Could you check a few things on this drawing? It's one solid part, dimensions in mm from its lowest x, y, z. A direction names the side the tool comes from. Round coordinates to 2 decimals unless told otherwise and drop trailing zeros. Loops run counter-clockwise (first coordinate to the right, second up) from the corner with the lowest first, then second, coordinate; pieces in that order, holes last. Notation, with made-up numbers: M 85.5,-24.5 L 132.5,-24.5 A10 cw 132.5,-10.5 Z; hole C 23,51 d1. An arc over 180 degrees is marked long. Write item = value, one per line. Start each with the question number.
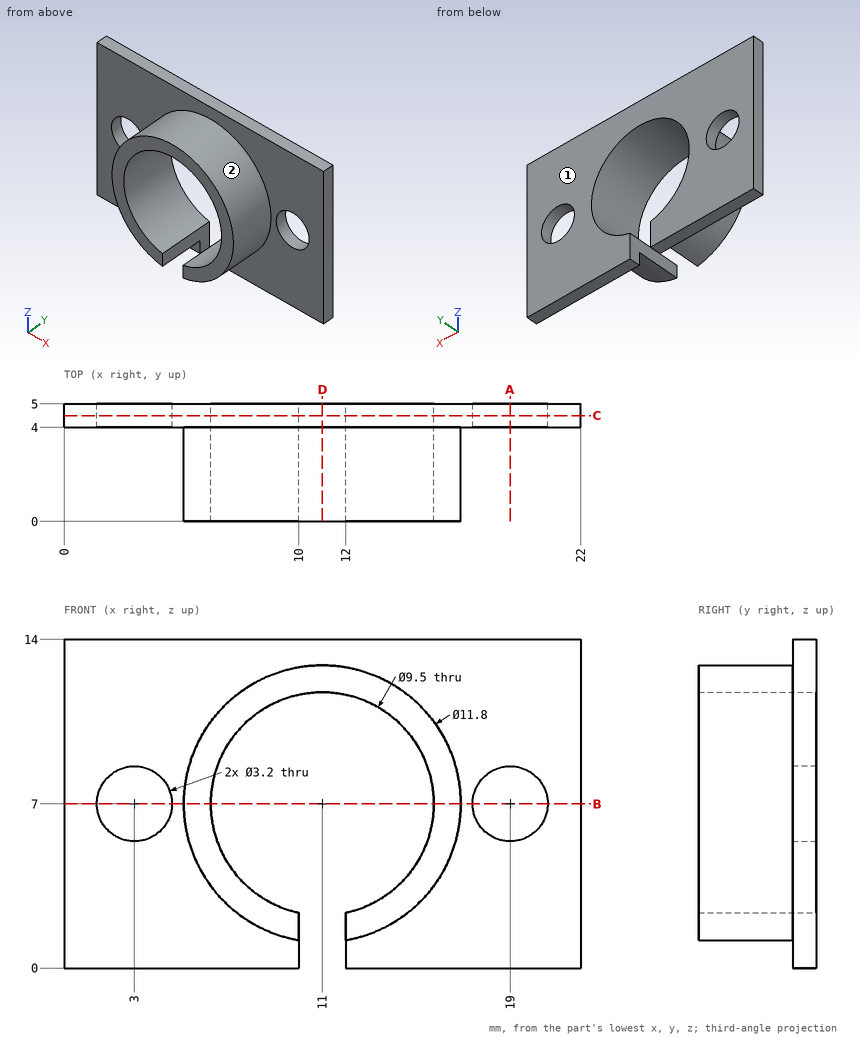
Item 1: For the marked faces 1 and 2, which set-ups out of +Z, -Z, +X, -X, +Y, -Y let a thin tool reach every point of the face, with its end or its side?
Item 2: I want a section at B-B, the plane z = 7. List the corners of the cut face in (x, y) for me.
Item 3: Please list where these lines run through material, in increasing order: line 1 (X direction, y = 4.85, z = 7); line 2 (X direction, y = 4.2, z = 5.75); line 3 (Y direction, x = 11, z = 13.5). Write a range as [from, to].
Item 4: I want a section at C-C, the plane y = 4.5. List the corners of the cut face in (x, z) for me, then the cut area to 3 significant figures.
Item 5: I want a section at D-D, the plane x = 11. List the corners of the cut face in (y, z) for me, then the cut area to 3 significant figures.
Item 6: Will these pins go through, and if not, where does the flat tip stop? pin 1 Ø1 at (x, z) = (18, 6) entering from +Y; pin 2 Ø1 at (x, z) = (4.5, 2) entering from -Y; pin 3 Ø2 at (y, z) = (1, 2.5) entering from -X; pin 4 Ø3 at (x, y) = (9, 2) entering from +Z.
Item 7: I want a section at A-A, the plane x = 19. List the corners of the cut face in (y, z) for me, then the cut area to 3 significant figures.
Worked out:
q1.face_1 = +Z, -Z, +X, -X, +Y
q1.face_2 = -Y
q2.outline = M 0,4 L 1.4,4 L 1.4,5 L 0,5 Z; M 4.6,4 L 5.1,4 L 5.1,0 L 6.25,0 L 6.25,5 L 4.6,5 Z; M 15.75,0 L 16.9,0 L 16.9,4 L 17.4,4 L 17.4,5 L 15.75,5 Z; M 20.6,4 L 22,4 L 22,5 L 20.6,5 Z
q3.line_1 = [0, 1.4], [4.6, 6.25], [15.75, 17.4], [20.6, 22]
q3.line_2 = [0, 2], [4, 6.42], [15.58, 18], [20, 22]
q3.line_3 = [4, 5]
q4.outline = M 0,0 L 10,0 L 10,2.36 A4.75 cw long 12,2.36 L 12,0 L 22,0 L 22,14 L 0,14 Z; hole C 3,7 d3.2; hole C 19,7 d3.2
q4.area = 216 mm2
q5.outline = M 0,11.75 L 5,11.75 L 5,14 L 4,14 L 4,12.9 L 0,12.9 Z
q5.area = 6.85 mm2
q6.pin_1 = 5
q6.pin_2 = 4
q6.pin_3 = 6.25
q6.pin_4 = 12.88
q7.outline = M 4,0 L 5,0 L 5,5.4 L 4,5.4 Z; M 4,8.6 L 5,8.6 L 5,14 L 4,14 Z
q7.area = 10.8 mm2
